```python
from build123d import *

# Parameters (mm, degrees)
BOSS_EXTRUDE1_DEPTH      = 15
BOSS_EXTRUDE2_DEPTH      = 15
BOSS_EXTRUDE3_DEPTH      = 19
BOSS_EXTRUDE3_DEPTH_BACK = 19
BOSS_EXTRUDE3_START      = -13.6
SKETCH9_W                = 25.65
SKETCH9_H                = 25.65
CUT_EXTRUDE2_DEPTH       = 41
SKETCH10_R               = 4
CUT_EXTRUDE3_DEPTH       = 41


with BuildPart() as part:
    # Sweep1: sweep along a path in Sketch1
    with BuildLine(Plane(origin=(0, 0, 0), x_dir=(1, 0, 0), z_dir=(0, 1, 0))) as sweep1_path:
        Line((21.279643058, 26.852704607), (21.279643058, 4.852704607))
        ThreePointArc((21.279643058, 4.852704607), (17.372739998, -11.11349039), (6.534906261, -23.471671247))
        Line((6.534906261, -23.471671247), (-11.486438713, -36.090352847))
    # Sketch5 → Sweep1 (sweep)
    with BuildSketch(Plane.XY.offset(-26.852704607)):
        Polygon((21.279643058, 9.6), (21.279643058, 0), (21.279643058, -9.6), (7.029643058, -9.6), (7.029643058, -13.6), (25.029643058, -13.6), (25.029643058, 13.6), (7.029643058, 13.6), (7.029643058, 9.6), align=None)
    sweep(path=sweep1_path.line)

    # Sketch6 → Boss-Extrude1 (add)
    with BuildSketch(Plane(origin=(0, 0, -26.852704607), x_dir=(-1, 0, 0), z_dir=(0, 0, -1))):
        Polygon((-7.029643058, 9.6), (-10.029643058, 8.1), (-10.029643058, 9.6), align=None)
        Polygon((-7.029643058, -9.6), (-10.029643058, -8.1), (-10.029643058, -9.6), align=None)
    extrude(amount=-BOSS_EXTRUDE1_DEPTH)

    # Sketch7 → Boss-Extrude2 (add)
    with BuildSketch(Plane(origin=(-24.66443519, 0, 17.270223446), x_dir=(0.5735764363510444, 0, 0.8191520442889931), z_dir=(-0.8191520442889931, 0, 0.5735764363510444))):
        Polygon((8.72513573, 9.6), (11.72513573, 8.1), (11.72513573, 9.6), align=None)
        Polygon((11.72513573, -8.1), (11.72513573, -9.6), (8.72513573, -9.6), align=None)
    extrude(amount=-BOSS_EXTRUDE2_DEPTH)

    # Sketch8 → Boss-Extrude3 (add, two sides: drawn at the far end of the back side and taken through both)
    with BuildSketch(Plane(origin=(0, 13.6, 0), x_dir=(1, 0, 0), z_dir=(0, 1, 0)).offset(BOSS_EXTRUDE3_START - BOSS_EXTRUDE3_DEPTH_BACK)):
        with BuildLine():
            Line((8.685817898, -26.543491413), (25.029643058, -26.543491413))
            Line((25.029643058, -26.543491413), (55.029643058, -26.543491413))
            Line((55.029643058, -26.543491413), (55.029643058, 4.852704607))
            Line((55.029643058, 4.852704607), (25.029643058, 4.852704607))
            ThreePointArc((25.029643058, 4.852704607), (20.699030623, -12.84504769), (8.685817898, -26.543491413))
        make_face()
    extrude(amount=BOSS_EXTRUDE3_DEPTH + BOSS_EXTRUDE3_DEPTH_BACK)

    # Sketch9 → Cut-Extrude2 (cut)
    with BuildSketch(Plane(origin=(0, 0, -4.852704607), x_dir=(-1, 0, 0), z_dir=(0, 0, -1))):
        with Locations((-42.204643058, 0)):
            Rectangle(SKETCH9_W, SKETCH9_H)
    extrude(amount=-CUT_EXTRUDE2_DEPTH, mode=Mode.SUBTRACT)

    # Sketch10 → Cut-Extrude3 (cut)
    with BuildSketch(Plane.XZ.offset(19)):
        with Locations(Location((42.779643058, 10.845393403, 0), (0, 0, 270))):
            Circle(SKETCH10_R)
    extrude(amount=-CUT_EXTRUDE3_DEPTH, mode=Mode.SUBTRACT)


solid = part.part
```
CAD build for the part. Positions are in the model's coordinates, mm. A direction names the side the tool comes from. Coordinates: 2 decimals unless noted, no trailing zeros. Order: outer loops, then holes, each group sorted by start corner. A loop starts at its lowest first (then second) coordinate and runs counter-clockwise, first axis right, second up. Notation, with made-up numbers: M 23,69.5 L 41,69.5 A22 cw 41,105.5 Z; hole C 15,78 d1. An arc over 180 degrees is marked long. Answer as CSV lines item,"result".
1) Cut at A-A (x = 50). List the corners of the cut face in (y, z) (1 decimal), then the cut area to 3 significant figures.
Verdict:
outline,"M -19,-4.9 L -12.8,-4.9 L -12.8,26.5 L -19,26.5 Z; M 12.8,-4.9 L 19,-4.9 L 19,26.5 L 12.8,26.5 Z"
area,"388 mm2"
2) Drill centre lines: L1, parallel to Y at x = 14, z = -19.5; L2, parallel to Z at x = 50.5, y = 17; L3, parallel to Y at x = 50.5, z = -1 (3 decimals). Where is each one in solid material? Low to high. Write a range as from..to.
Verdict:
L1,"-13.6..-9.6, 9.6..13.6"
L2,"-4.85..26.54"
L3,"-19..-12.825, 12.825..19"
3) Flat gauge pins, fed straight in: P1, Ø5, axis at y = 8.5, z = 22, coming from the +X side; P2, Ø4, axis at x = 3.5, y = 7, coming from the +Z side; P3, Ø15.5, axis at y = -2, z = -21.5, coming from the -X side; P4, Ø7.5, axis at x = 44.5, z = 13.5, coming from the +Y side. Where does each tip first touch, or does it go through?
Verdict:
P1,"x = 29.38"
P2,"z = 31.58"
P3,"x = 7.03"
P4,"y = 19"
4) Cut at B-B (y = 10.5). List the corners of the cut face in (x, z), then the cut area to 3 significant figures.
Verdict:
outline,"M -19.66,24.42 L -1.64,11.8 A20.33 cw 7.03,-4.85 L 7.03,-26.85 L 25.03,-26.85 L 25.03,-4.85 L 29.38,-4.85 L 29.38,26.54 L 8.69,26.54 L -9.34,39.16 Z"
area,"1,590 mm2"
5) Mould opens along Y. For faces 6 (the flat face through (-6.142, 9.194, 17.571)), 7 (the cylindrical face through (5, -12, 4)), 8 (the flat face through (8, 13.6, 7)) say: released by +Y, released by -Y, zero draft, split by the parting line, or undercut.
Verdict:
face 6,"undercut"
face 7,"zero draft"
face 8,"released by +Y"
6) Cut at D-D (x = -4.5). List the corners of the cut face in (y, z), then the cut area to 3 significant figures.
Verdict:
outline,"M -13.6,13.8 L -9.6,13.8 L -9.6,31.2 L 9.6,31.2 L 9.6,13.8 L 13.6,13.8 L 13.6,35.78 L -13.6,35.78 Z"
area,"264 mm2"
7) Cut at C-C (z = -22). List the corners of the cut face in (x, y).
Verdict:
outline,"M 7.03,-13.6 L 25.03,-13.6 L 25.03,13.6 L 7.03,13.6 L 7.03,9.6 L 10.03,8.1 L 10.03,9.6 L 21.28,9.6 L 21.28,-9.6 L 10.03,-9.6 L 10.03,-8.1 L 7.03,-9.6 Z"
8) 3-axis set-ups, long thin cutter, end or side, ignore diameter. For faces 1 (the cylindrical face through (20.817, -16.338, 12.616)), 2 (the flat face through (25.03, 0, -16)), 3 (the flat face through (29.38, 0, 11)), 4 (the flat face through (26, 0, 26.543)), 5 (the flat face through (7.03, 12, -16)): which of +Z, -Z, +X, -X, +Y, -Y reach the whole face in a straight line?
Verdict:
face 1,"-Z, -X, -Y"
face 2,"-Z, +X, +Y, -Y"
face 3,"+Z, -Z, +X"
face 4,"+Z, +X, +Y, -Y"
face 5,"-Z, -X, +Y, -Y"
